from build123d import *

# Parameters (mm, degrees)
BOSS_EXTRUDE1_DEPTH = 140
BOSS_EXTRUDE2_DEPTH = 162.5
CUT_EXTRUDE1_DEPTH  = 100
SKETCH4_R           = 7
CUT_EXTRUDE2_DEPTH  = 1000
SKETCH5_R           = 2.5
CUT_EXTRUDE3_DEPTH  = 1000


with BuildPart() as part:
    # Sketch1 → Boss-Extrude1 (new body)
    with BuildSketch(Plane.XY):
        Polygon((-148.823444479, 16.363961031), (-134.823444479, 16.363961031), (-134.823444479, 6.363961031), (-134.823444479, 5.363961031), (-129.823444479, 5.363961031), (-129.823444479, 6.363961031), (-111.771895875, 6.363961031), (-105.407934844, 0), (-105.307934844, 0), (-98.943973814, 6.363961031), (-50.443973814, 6.363961031), (-44.080012783, 0), (-44.080012783, -1), (-40.080012783, -1), (-40.080012783, 0), (-33.716051752, 6.363961031), (-32.716051752, 6.363961031), (-32.716051752, 16.363961031), (-20.216051752, 16.363961031), (-20.216051752, 5.363961031), (-15.216051752, 5.363961031), (-15.216051752, 6.363961031), (13.676555521, 6.363961031), (13.676555521, -9.636038969), (-148.823444479, -9.636038969), align=None)
    extrude(amount=BOSS_EXTRUDE1_DEPTH)

    # Sketch2 → Boss-Extrude2 (add)
    with BuildSketch(Plane(origin=(13.676555521, 0, 0), x_dir=(0, 0, -1), z_dir=(1, 0, 0))):
        Polygon((-86.25, -11.136038969), (-93.75, -18.636038969), (-46.25, -18.636038969), (-53.75, -11.136038969), (-31, -11.136038969), (-31, -8.713113528), (-109, -8.713113528), (-109, -11.136038969), align=None)
    extrude(amount=-BOSS_EXTRUDE2_DEPTH)

    # Sketch3 → Cut-Extrude1 (cut)
    with BuildSketch(Plane.XZ.offset(9.636038969)):
        with BuildLine():
            Line((-121.342924919, 0), (-41.039209534, 0))
            Line((-41.039209534, 0), (-41.039209534, 25))
            ThreePointArc((-41.039209534, 25), (-42.503675628, 28.535533906), (-46.039209534, 30))
            Line((-46.039209534, 30), (-116.342924919, 30))
            ThreePointArc((-116.342924919, 30), (-119.878458825, 28.535533906), (-121.342924919, 25))
            Line((-121.342924919, 25), (-121.342924919, 0))
        make_face()
        with BuildLine():
            Line((-121.342924919, 140), (-41.039209534, 140))
            Line((-41.039209534, 140), (-41.039209534, 115))
            ThreePointArc((-41.039209534, 115), (-42.503675628, 111.464466094), (-46.039209534, 110))
            Line((-46.039209534, 110), (-116.342924919, 110))
            ThreePointArc((-116.342924919, 110), (-119.878458825, 111.464466094), (-121.342924919, 115))
            Line((-121.342924919, 115), (-121.342924919, 140))
        make_face()
    extrude(amount=-CUT_EXTRUDE1_DEPTH, mode=Mode.SUBTRACT)

    # Sketch4 → Cut-Extrude2 (cut)
    with BuildSketch(Plane(origin=(13.676555521, 0, 0), x_dir=(0, 0, -1), z_dir=(1, 0, 0))):
        with Locations((-70, -9.636038969)):
            Circle(SKETCH4_R)
    extrude(amount=-CUT_EXTRUDE2_DEPTH, mode=Mode.SUBTRACT)

    # Sketch5 → Cut-Extrude3 (cut)
    with BuildSketch(Plane(origin=(13.676555521, 0, 0), x_dir=(0, 0, -1), z_dir=(1, 0, 0))):
        with Locations((-92, 0.863961031)):
            Circle(SKETCH5_R)
        with Locations((-48, 0.863961031)):
            Circle(SKETCH5_R)
    extrude(amount=-CUT_EXTRUDE3_DEPTH, mode=Mode.SUBTRACT)


solid = part.part
Verification items for the finished model (mm, model axes). A direction names the side the tool comes from. Give positions to 0.01 mm unless a question says otherwise; leave off trailing zeros. Loops run counter-clockwise (first coordinate to the right, second up) from the corner with the lowest first, then second, coordinate; pieces in that order, holes last. Notation, with made-up numbers: (21.25, 61.5) - (50.25, 61.5) arc R31 cw to (50.25, 87.5) - close; hole circle Ø5 at (79, 23). An arc over 180 degrees is marked (long way). Write each question's results on one line, items separated by ' | '.
1) Sectioned sample at C-C on x = -66. Record the boundary of the cut face in (y, z), plus the area to 3 significant figures.
Solution:
outline: (-18.64, 46.25) - (-11.14, 53.75) - (-11.14, 31) - (-9.64, 31) - (-9.64, 30) - (6.36, 30) - (6.36, 110) - (-9.64, 110) - (-9.64, 109) - (-11.14, 109) - (-11.14, 86.25) - (-18.64, 93.75) - close; hole circle Ø14 at (-9.64, 70); hole circle Ø5 at (0.86, 48); hole circle Ø5 at (0.86, 92) | area: 1,500 mm2
2) Mould release check, pull along X, two halves, no side actions. Record for faces 1 (the flat face through (-13, 1, 140)), 2 (the cylindrical face through (-42.47, -5.21, 111.5)), 3 (the flat face through (-41.039, -5, 128)), 4 (the flat face through (13.677, 0, 71)): pulls with the +X half, pulls with the -X half, needs draft (parallel to the pull), parting line crosses it, or undercut.
Solution:
face 1: needs draft | face 2: undercut | face 3: undercut | face 4: pulls with the +X half
3) Sectioned sample at A-A on z = 70. Record the boundary of the cut face in (x, y), plus the area to 3 significant figures.
Solution:
outline: (-148.82, -18.64) - (13.68, -18.64) - (13.68, -16.64) - (-148.82, -16.64) - close; (-148.82, -2.64) - (13.68, -2.64) - (13.68, 6.36) - (-15.22, 6.36) - (-15.22, 5.36) - (-20.22, 5.36) - (-20.22, 16.36) - (-32.72, 16.36) - (-32.72, 6.36) - (-33.72, 6.36) - (-40.08, 0) - (-40.08, -1) - (-44.08, -1) - (-44.08, 0) - (-50.44, 6.36) - (-98.94, 6.36) - (-105.31, 0) - (-105.41, 0) - (-111.77, 6.36) - (-129.82, 6.36) - (-129.82, 5.36) - (-134.82, 5.36) - (-134.82, 16.36) - (-148.82, 16.36) - close | area: 1,930 mm2
4) Sectioned sample at B-B on y = -4.5. Record the boundary of the cut face in (x, z), plus the area to 3 significant figures.
Solution:
outline: (-148.82, 0) - (-121.34, 0) - (-121.34, 25) arc R5 cw to (-116.34, 30) - (-46.04, 30) arc R5 cw to (-41.04, 25) - (-41.04, 0) - (13.68, 0) - (13.68, 65.24) - (-148.82, 65.24) - close; (-148.82, 74.76) - (13.68, 74.76) - (13.68, 140) - (-41.04, 140) - (-41.04, 115) arc R5 cw to (-46.04, 110) - (-116.34, 110) arc R5 cw to (-121.34, 115) - (-121.34, 140) - (-148.82, 140) - close | area: 16,400 mm2
5) Tool access check on faces 5 (the flat face through (-134.823, 11, 69)), 6 (the cylindrical face through (-119.839, -1.748, 111.426)), 7 (the flat face through (-121.343, -2, 13)). Record the directions out of +Z, -Z, +X, -X, +Y, -Y that give a thin tool (end or side, any length) a straight path to the whole face; none if there is none.
Solution:
face 5: +Z, -Z, +Y | face 6: +Z, +Y, -Y | face 7: -Z, +Y, -Y
6) Depth check by flat-ended pin: P1, Ø0.8, axis at x = -84, y = -10, coming from the +Z side; P2, Ø4.5, axis at x = -41, z = 16.5, coming from the +Y side; P3, Ø1.5, axis at x = -18.5, z = 84, coming from the +Y side. Enter the tip coordinate at first touch or a pass-through.
Solution:
P1: z = 110 | P2: y = 1.33 | P3: y = 5.36
7) Material ranges on L1, parallel to Z at x = -109, y = 0; L2, parallel to X at y = 6.5, z = 47.5; L3, parallel to Y at x = -66.5, z = 92, recorded low to high. Write a range as from..to.
Solution:
L1: 30..45.65, 50.35..89.65, 94.35..110 | L2: -148.82..-134.82, -32.72..-20.22 | L3: -18.64..-16.89, -11.14..-1.64, 3.36..6.36
